Could you check a few things on this drawing? It's one solid part, dimensions in mm from its lowest x, y, z. Give positions to 0.01 mm unless a question says otherwise; leave off trailing zeros. Order: outer loops, then holes, each group sorted by start corner. A loop starts at its lowest first (then second) coordinate and runs counter-clockwise, first axis right, second up. Notation, with made-up numbers: (53, 68.25) - (102, 68.25) arc R8 ccw to (102, 77.25) - close; hole circle Ø3 at (-32, -28). An arc over 180 degrees is marked (long way). Answer as CSV lines item,"result".
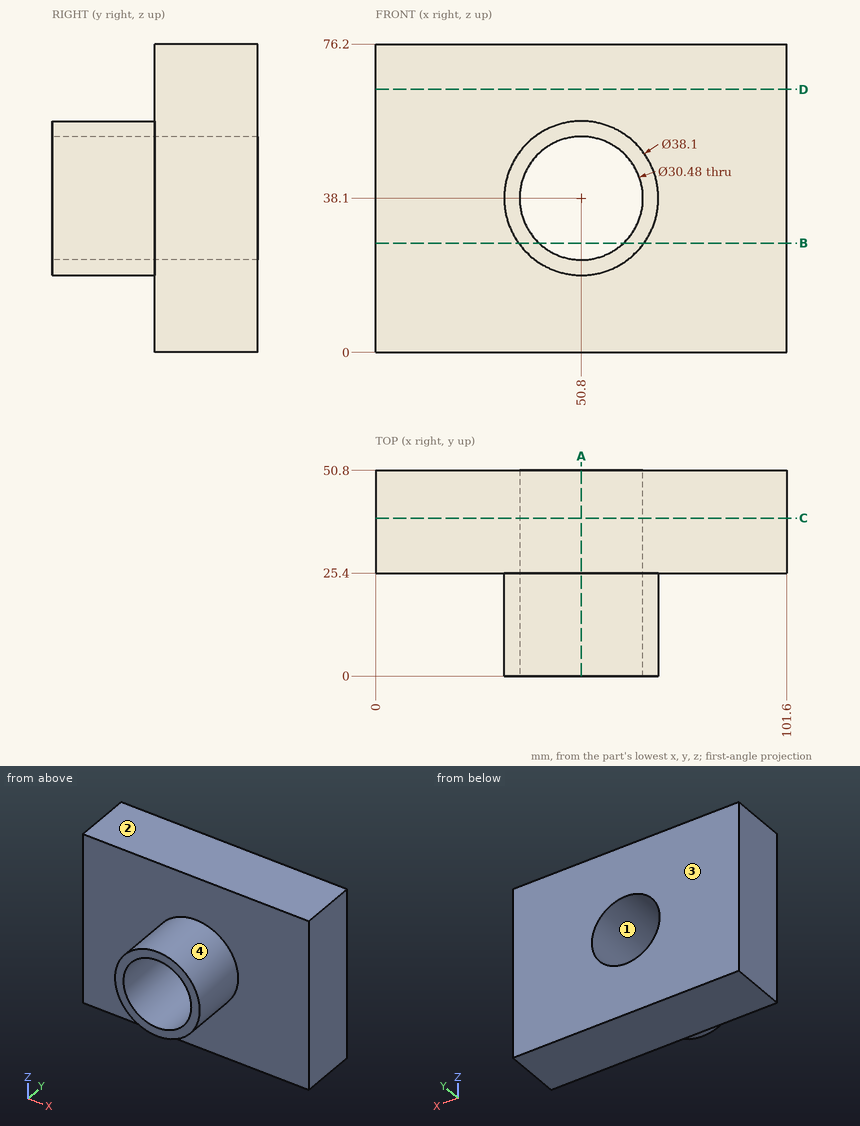
1) I want a section at B-B on z = 27. Write out the boundary of the cut face in (x, y).
Answer block:
outline,"(0, 25.4) - (35.32, 25.4) - (35.32, 0) - (40.36, 0) - (40.36, 50.8) - (0, 50.8) - close; (61.24, 0) - (66.28, 0) - (66.28, 25.4) - (101.6, 25.4) - (101.6, 50.8) - (61.24, 50.8) - close"
2) I need wall thicknesses on line 1 along Z through (x, y) = (50.8, 22); line 2 along Z through (x, y) = (50.8, 34); line 3 along Y through (x, z) = (72.5, 18). Which ranges of each line are inside material? Lowest first, please. Write a range as [from, to].
Answer block:
line 1,"[19.05, 22.86], [53.34, 57.15]"
line 2,"[0, 22.86], [53.34, 76.2]"
line 3,"[25.4, 50.8]"
3) I want a section at D-D on z = 65. Write out the boundary of the cut face in (x, y), plus the area to 3 significant figures.
Answer block:
outline,"(0, 25.4) - (101.6, 25.4) - (101.6, 50.8) - (0, 50.8) - close"
area,"2,580 mm2"
4) I want a section at A-A on x = 50.8. Write out the boundary of the cut face in (y, z), plus the area to 3 significant figures.
Answer block:
outline,"(0, 19.05) - (25.4, 19.05) - (25.4, 0) - (50.8, 0) - (50.8, 22.86) - (0, 22.86) - close; (0, 53.34) - (50.8, 53.34) - (50.8, 76.2) - (25.4, 76.2) - (25.4, 57.15) - (0, 57.15) - close"
area,"1,350 mm2"
5) I want a section at C-C on y = 39. Write out the boundary of the cut face in (x, z).
Answer block:
outline,"(0, 0) - (101.6, 0) - (101.6, 76.2) - (0, 76.2) - close; hole circle Ø30.48 at (50.8, 38.1)"
6) If we mould it in two halves opening along Z, with no side actions, what happens to the marked faces 1, 2, 3 and 4? For each: +Z half, -Z half, draft (parallel to the pull), parting line (faces both ways), or undercut.
Answer block:
face 1,"undercut"
face 2,"+Z half"
face 3,"draft"
face 4,"parting line"
7) I'm going to push a flat-ended pin straight in: P1, Ø12, axis at y = 14.5, z = 17.5, coming from the -X side. Where does the tip first touch, or does it pass through?
Answer block:
P1,"x = 38.56"
